The model under review builds one solid part; all positions refer to its coordinate system, in mm. A direction names the side the tool comes from. Coordinates: 2 decimals unless noted, no trailing zeros. Write each loop counter-clockwise with the first axis right and the second up, starting at its lowest first coordinate (ties: lowest second). Pieces come first, ordered by that corner, then holes. Notation, with made-up numbers: (-7, 24.25) -> (33, 24.25) arc R13 cw to (33, 40.25) -> close; hole circle Ø5 at (-2.75, -6.5). An arc over 180 degrees is marked (long way). Write each question's results on one line, items separated by ' | '.
```python
from build123d import *

# Parameters (mm, degrees)
EXTRUDE_1_DEPTH     = 4
SKETCH_2_R          = 1.5
CUT_EXTRUDE_1_DEPTH = 4
SKETCH_3_R          = 1.5
CUT_EXTRUDE_2_DEPTH = 4
EXTRUDE_2_DEPTH     = 4
FILLET_2_R          = 3
SKETCH_6_R          = 1.5
CUT_EXTRUDE_3_DEPTH = 167.255826966


with BuildPart() as part:
    # 草图1 → 凸台-拉伸1 (new body)
    with BuildSketch(Plane(origin=(0, 0, 0), x_dir=(1, 0, 0), z_dir=(0, 1, 0))):
        Polygon((0, 0), (60, 0), (60, 155), (-30, 155), (-30, 120), (0, 90), align=None)
    extrude(amount=EXTRUDE_1_DEPTH)

    # 草图2 → 切除-拉伸1 (cut)
    with BuildSketch(Plane(origin=(0, 4, 0), x_dir=(1, 0, 0), z_dir=(0, 1, 0))):
        with Locations(Location((45, 25, 0), (0, 0, 270))):
            Circle(SKETCH_2_R)
        with Locations(Location((21, 25, 0), (0, 0, 270))):
            Circle(SKETCH_2_R)
        with Locations(Location((45, 55, 0), (0, 0, 270))):
            Circle(SKETCH_2_R)
        with Locations(Location((21, 55, 0), (0, 0, 270))):
            Circle(SKETCH_2_R)
    extrude(amount=-CUT_EXTRUDE_1_DEPTH, mode=Mode.SUBTRACT)

    # 草图3 → 切除-拉伸2 (cut)
    with BuildSketch(Plane(origin=(0, 4, 0), x_dir=(1, 0, 0), z_dir=(0, 1, 0))):
        with Locations(Location((30, 147.590674679, 0), (0, 0, 270))):
            Circle(SKETCH_3_R)
        with Locations(Location((43, 147.590674679, 0), (0, 0, 270))):
            Circle(SKETCH_3_R)
        with Locations(Location((-13, 147.590674679, 0), (0, 0, 90))):
            Circle(SKETCH_3_R)
        with Locations(Location((0, 147.590674679, 0), (0, 0, 90))):
            Circle(SKETCH_3_R)
    extrude(amount=-CUT_EXTRUDE_2_DEPTH, mode=Mode.SUBTRACT)

    # 草图5 → 凸台-拉伸2 (add)
    with BuildSketch(Plane(origin=(0, 4, 0), x_dir=(1, 0, 0), z_dir=(0, 1, 0))):
        Polygon((0, 0), (-10, 0), (-10, 100), (0, 90), align=None)
    extrude(amount=-EXTRUDE_2_DEPTH)

    # 圆角2
    fillet_2_edges = [part.edges().sort_by_distance(p)[0] for p in [
        (-30, 2, -120),
        (-30, 2, -155),
        (60, 2, -155),
        (60, 2, 0),
        (-10, 2, 0),
        (-10, 2, -100),
    ]]
    fillet(fillet_2_edges, radius=FILLET_2_R)

    # 草图6 → 切除-拉伸3 (cut, through all)
    with BuildSketch(Plane(origin=(0, 4, 0), x_dir=(1, 0, 0), z_dir=(0, 1, 0))):
        with Locations(Location((7.5, 8, 0), (0, 0, 270))):
            Circle(SKETCH_6_R)
        with Locations(Location((42.5, 8, 0), (0, 0, 270))):
            Circle(SKETCH_6_R)
    extrude(amount=-CUT_EXTRUDE_3_DEPTH, mode=Mode.SUBTRACT)


solid = part.part
```
Q1. Draft analysis for pull direction Z (two halves, no side actions). For faces 3 (the cylindrical face through (59.1, 2.03, -154.14)), 4 (the cylindrical face through (22.265, 2.028, -54.194)), 5 (the flat face through (-20, 2, -110)), state which applies: pulls with the +Z half, pulls with the -Z half, needs draft (parallel to the pull), parting line crosses it, or undercut.
Solution:
face 3: pulls with the -Z half | face 4: undercut | face 5: pulls with the +Z half
Q2. Add section B-B (y = 2.05). Count the separate pieces of the cut face and the enclosed holes in it, plus the area to 3 significant figures.
Solution:
separate pieces: 1 | enclosed holes: 10 | area: 11,700 mm²
Q3. Machinability: for faces 1 (the cylindrical face through (43.67, 2.03, -54.31)), 2 (the flat face through (-10, 2, -50)), which of the approach directions +Z, -Z, +X, -X, +Y, -Y give a long, thin tool a straight path to every point of the face, cutting with its end or side? Answer none if there is none.
Solution:
face 1: +Y, -Y | face 2: +Z, -X, +Y, -Y
Q4. For line 1 (X direction, y = 0.95, z = -55); line 2 (Z direction, x = 46, y = 1.5); line 3 (X direction, y = 3.65, z = -95.5), list the stretches that pass through material, from the lowest coordinate up. Write a range as from..to.
Solution:
line 1: -10..19.5, 22.5..43.5, 46.5..60 | line 2: -155..-56.12, -53.88..-26.12, -23.88..0 | line 3: -10..60
Q5. Add section A-A (x = 30). Write out the cut boundary in (y, z).
Solution:
outline: (0, -155) -> (4, -155) -> (4, -149.09) -> (0, -149.09) -> close; (0, -146.09) -> (4, -146.09) -> (4, 0) -> (0, 0) -> close
Q6. Add section C-C (x = 21). Write out the cut boundary in (y, z).
Solution:
outline: (0, -155) -> (4, -155) -> (4, -56.5) -> (0, -56.5) -> close; (0, -53.5) -> (4, -53.5) -> (4, -26.5) -> (0, -26.5) -> close; (0, -23.5) -> (4, -23.5) -> (4, 0) -> (0, 0) -> close
Q7. Clearance check with a flat-ended pin moving along its axis: P1, Ø2, axis at y = 1.5, z = -33, coming from the -X side. State where the tip first meets the part, or that it passes through.
Solution:
P1: x = -10
Q8. Add section D-D (z = -55). Write out the cut boundary in (x, y).
Solution:
outline: (-10, 0) -> (19.5, 0) -> (19.5, 4) -> (-10, 4) -> close; (22.5, 0) -> (43.5, 0) -> (43.5, 4) -> (22.5, 4) -> close; (46.5, 0) -> (60, 0) -> (60, 4) -> (46.5, 4) -> close
